from build123d import *

# Parameters (mm, degrees)
SKETCH1_W                  = 173.0375
SKETCH1_H                  = 114.3
BOSS_EXTRUDE1_DEPTH        = 3.175
SKETCH3_R                  = 3.175
SKETCH3_R_2                = 3.7703125
CUT_EXTRUDE1_DEPTH         = 149.360729792
F_6_CLEARANCE_HOLE1_D      = 4.3053
F_3_0_213_DIAMETER_HOLE1_D = 5.4102
F_1_4_CLEARANCE_HOLE1_D    = 7.14248
CUT_EXTRUDE5_REACH         = 150.361
SKETCH16_R                 = 1.190625
CUT_EXTRUDE6_DEPTH         = 149.360729792
FILLET5_R                  = 3.175
FILLET6_R                  = 3.175
FILLET7_R                  = 2.54


with BuildPart() as part:
    # Sketch1 → Boss-Extrude1 (new body)
    with BuildSketch(Plane.XY):
        with Locations((25.118, -40.513)):
            Rectangle(SKETCH1_W, SKETCH1_H)
    extrude(amount=BOSS_EXTRUDE1_DEPTH)

    # Sketch3 → Cut-Extrude1 (cut, through all)
    with BuildSketch(Plane.XY.offset(3.175)):
        with Locations((100.302, -26.543)):
            Circle(SKETCH3_R)
        with Locations((99.413, -51.6255)):
            Circle(SKETCH3_R_2)
        with Locations((-47.907, -51.6255)):
            Circle(SKETCH3_R_2)
        with Locations((-47.907, -6.5405)):
            Circle(SKETCH3_R_2)
    extrude(amount=-CUT_EXTRUDE1_DEPTH, mode=Mode.SUBTRACT)

    # #6 Clearance Hole1 (through all)
    with Locations(Plane.XY.offset(3.175)):
        with Locations((18.387, 10.287), (-56.162, -40.894), (106.398, -40.894), (18.387, -91.313)):
            Hole(F_6_CLEARANCE_HOLE1_D / 2)

    # #3 (0.213) Diameter Hole1 (through all)
    with Locations(Plane(origin=(18.387, 10.287, 3.175), x_dir=(1, 0, 0), z_dir=(0, 0, 1))):
        with Locations((0, 0), (-74.549, -51.181), (0, -101.6), (88.011, -51.181)):
            Hole(F_3_0_213_DIAMETER_HOLE1_D / 2)

    # 1/4 Clearance Hole1 (through all)
    with Locations(Plane(origin=(0, 0, 0), x_dir=(-1, 0, 0), z_dir=(0, 0, -1))):
        with Locations((-102.7785, 10.287), (52.5425, 10.287)):
            Hole(F_1_4_CLEARANCE_HOLE1_D / 2)

    # Sketch16 → Cut-Extrude5 (cut, up to next)
    with BuildSketch(Plane(origin=(0, 0, 0), x_dir=(-1, 0, 0), z_dir=(0, 0, -1)), mode=Mode.PRIVATE) as cut_extrude5_sk1:
        with Locations((-98.142490655, -57.489441166)):
            Circle(SKETCH16_R)
    cut_extrude5_tool1 = extrude(cut_extrude5_sk1.sketch, amount=-CUT_EXTRUDE5_REACH, mode=Mode.PRIVATE) & part.part
    # Sketch16 → Cut-Extrude5 (cut, up to next)
    with BuildSketch(Plane(origin=(0, 0, 0), x_dir=(-1, 0, 0), z_dir=(0, 0, -1)), mode=Mode.PRIVATE) as cut_extrude5_sk2:
        with Locations((49.177509345, -57.489441166)):
            Circle(SKETCH16_R)
    cut_extrude5_tool2 = extrude(cut_extrude5_sk2.sketch, amount=-CUT_EXTRUDE5_REACH, mode=Mode.PRIVATE) & part.part
    # Sketch16 → Cut-Extrude5 (cut, up to next)
    with BuildSketch(Plane(origin=(0, 0, 0), x_dir=(-1, 0, 0), z_dir=(0, 0, -1)), mode=Mode.PRIVATE) as cut_extrude5_sk3:
        with Locations((49.177509345, -12.404441166)):
            Circle(SKETCH16_R)
    cut_extrude5_tool3 = extrude(cut_extrude5_sk3.sketch, amount=-CUT_EXTRUDE5_REACH, mode=Mode.PRIVATE) & part.part
    add(cut_extrude5_tool1.solids().sort_by_distance((98.142491, -57.489441, 0))[0], mode=Mode.SUBTRACT)
    add(cut_extrude5_tool2.solids().sort_by_distance((-49.177509, -57.489441, 0))[0], mode=Mode.SUBTRACT)
    add(cut_extrude5_tool3.solids().sort_by_distance((-49.177509, -12.404441, 0))[0], mode=Mode.SUBTRACT)

    # Sketch17 → Cut-Extrude6 (cut, through all)
    with BuildSketch(Plane(origin=(0, 0, 0), x_dir=(-1, 0, 0), z_dir=(0, 0, -1))):
        Polygon((-89.41175, 10.287), (-59.68051, 10.287), (-59.68051, 14.25702), (-52.53549, 14.25702), (-52.53549, 10.287), (-34.28051, 10.287), (-34.28051, 14.25702), (-27.13549, 14.25702), (-27.13549, 10.287), (-24.737, 10.287), (-24.737, 5.5245), (-12.037, 5.5245), (-12.037, 10.287), (42.35075, 10.287), (42.35075, 5.5245), (48.70075, 5.5245), (48.70075, 0.762), (55.05075, 0.762), (55.05075, -36.1315), (48.2245, -36.1315), (48.2245, -45.26026), (56.63825, -45.26026), (56.63825, -91.313), (22.39451, -91.313), (22.39451, -94.488), (15.24949, -94.488), (15.24949, -91.313), (-12.037, -91.313), (-12.037, -86.5505), (-24.737, -86.5505), (-24.737, -91.313), (-70.36175, -91.313), (-70.36175, -94.488), (-92.58675, -94.488), (-92.58675, -89.7255), (-106.87425, -89.7255), (-106.87425, -45.26026), (-100.048, -45.26026), (-100.048, -36.1315), (-106.87425, -36.1315), (-106.87425, -28.194), (-109.22375, -28.194), (-109.22375, -23.4315), (-106.87425, -23.4315), (-106.87425, 0), (-99.72923, 0), (-99.72923, 3.175), (-89.41175, 3.175), align=None)
    extrude(amount=-CUT_EXTRUDE6_DEPTH, mode=Mode.SUBTRACT)

    # Fillet5
    # the kernel refuses this fillet: 3.175 mm, written as the material it adds along each edge
    with BuildSketch(Plane(origin=(106.87425, 0, 0), x_dir=(0, -1, 0), z_dir=(0, 0, 1)), Plane(origin=(106.87425, -45.26026, 0), x_dir=(0, -1, 0), z_dir=(0, 0, 1)), Plane(origin=(106.87425, -36.1315, 0), x_dir=(-1, 0, 0), z_dir=(0, 0, 1)), Plane(origin=(106.87425, -89.7255, 0), x_dir=(-1, 0, 0), z_dir=(0, 0, 1)), Plane(origin=(92.58675, -94.488, 0), x_dir=(-1, 0, 0), z_dir=(0, 0, 1)), Plane(origin=(70.36175, -94.488, 0), x_dir=(0, 1, 0), z_dir=(0, 0, 1)), Plane(origin=(24.737, -91.313, 0), x_dir=(0, 1, 0), z_dir=(0, 0, 1)), Plane(origin=(12.037, -91.313, 0), x_dir=(-1, 0, 0), z_dir=(0, 0, 1)), Plane(origin=(-15.24949, -94.488, 0), x_dir=(-1, 0, 0), z_dir=(0, 0, 1)), Plane(origin=(-22.39451, -94.488, 0), x_dir=(0, 1, 0), z_dir=(0, 0, 1)), Plane(origin=(-56.63825, -91.313, 0), x_dir=(0, 1, 0), z_dir=(0, 0, 1)), Plane(origin=(-55.05075, -36.1315, 0), x_dir=(0, 1, 0), z_dir=(0, 0, 1)), Plane(origin=(-56.63825, -45.26026, 0), x_dir=(1, 0, 0), z_dir=(0, 0, 1)), Plane(origin=(-55.05075, 0.762, 0), x_dir=(1, 0, 0), z_dir=(0, 0, 1)), Plane(origin=(-48.70075, 5.5245, 0), x_dir=(1, 0, 0), z_dir=(0, 0, 1)), Plane(origin=(-42.35075, 10.287, 0), x_dir=(1, 0, 0), z_dir=(0, 0, 1)), Plane(origin=(12.037, 10.287, 0), x_dir=(0, -1, 0), z_dir=(0, 0, 1)), Plane(origin=(34.28051, 14.25702, 0), x_dir=(0, -1, 0), z_dir=(0, 0, 1)), Plane(origin=(27.13549, 14.25702, 0), x_dir=(1, 0, 0), z_dir=(0, 0, 1)), Plane(origin=(52.53549, 14.25702, 0), x_dir=(1, 0, 0), z_dir=(0, 0, 1)), Plane(origin=(59.68051, 14.25702, 0), x_dir=(0, -1, 0), z_dir=(0, 0, 1))) as fillet5_piece_1:
        with BuildLine():
            CenterArc((FILLET5_R, -FILLET5_R), FILLET5_R, 90, 90)
            Line((0, -FILLET5_R), (-FILLET5_R * 0.02, -FILLET5_R))
            Line((-FILLET5_R * 0.02, -FILLET5_R), (-FILLET5_R * 0.02, FILLET5_R * 0.02))
            Line((-FILLET5_R * 0.02, FILLET5_R * 0.02), (FILLET5_R, FILLET5_R * 0.02))
            Line((FILLET5_R, FILLET5_R * 0.02), (FILLET5_R, 0))
        make_face()
    extrude(amount=3.175)
    with BuildSketch(Plane(origin=(24.737, 10.287, 0), x_dir=(1, 0, 0), z_dir=(0, 0, 1))) as fillet5_piece_2:
        with BuildLine():
            CenterArc((3.175, -3.07858039), FILLET5_R, 104.15642815, 75.84357185)
            Line((0, -3.07858039), (-0.0635, -3.07858039))
            Line((-0.0635, -3.07858039), (-0.0635, 0))
            Line((-0.0635, 0), (0, 0.0635))
            ThreePointArc((0, 0.0635), (1.199245, 0.0635), (2.3829598, 0.061571608))
            Line((2.3829598, 0.061571608), (2.39849, 0))
        make_face()
    extrude(amount=3.175)
    with BuildSketch(Plane(origin=(89.41175, 10.287, 0), x_dir=(-1, 0, 0), z_dir=(0, 0, 1))) as fillet5_piece_3:
        with BuildLine():
            CenterArc((FILLET5_R, FILLET5_R), FILLET5_R, 180, 90)
            Line((0, FILLET5_R), (-FILLET5_R * 0.02, FILLET5_R))
            Line((-FILLET5_R * 0.02, FILLET5_R), (-FILLET5_R * 0.02, -FILLET5_R * 0.02))
            Line((-FILLET5_R * 0.02, -FILLET5_R * 0.02), (FILLET5_R, -FILLET5_R * 0.02))
            Line((FILLET5_R, -FILLET5_R * 0.02), (FILLET5_R, 0))
        make_face()
    extrude(amount=3.175)
    # the kernel refuses this fillet: 3.175 mm, written as the material it takes off along each edge
    with BuildSketch(Plane(origin=(99.72923, 0, -7.9375), x_dir=(1, 0, 0), z_dir=(0, 0, 1)), Plane(origin=(89.41175, 3.175, -7.9375), x_dir=(1, 0, 0), z_dir=(0, 0, 1))) as fillet5_2_piece_1:
        with BuildLine():
            CenterArc((FILLET5_R, FILLET5_R), FILLET5_R, 180, 90)
            Line((0, FILLET5_R), (-FILLET5_R * 0.02, FILLET5_R))
            Line((-FILLET5_R * 0.02, FILLET5_R), (-FILLET5_R * 0.02, -FILLET5_R * 0.02))
            Line((-FILLET5_R * 0.02, -FILLET5_R * 0.02), (FILLET5_R, -FILLET5_R * 0.02))
            Line((FILLET5_R, -FILLET5_R * 0.02), (FILLET5_R, 0))
        make_face()
    extrude(amount=19.05, mode=Mode.SUBTRACT)
    with BuildSketch(Plane(origin=(106.87425, -23.4315, -7.664518392), x_dir=(1, 0, 0), z_dir=(0, 0, 1))) as fillet5_2_piece_2:
        with BuildLine():
            CenterArc((3.175, 3.065807357), FILLET5_R, 180, 74.929937855)
            Line((0, 3.065807357), (-0.0635, 3.065807357))
            Line((-0.0635, 3.065807357), (-0.0635, 0))
            Line((-0.0635, 0), (0, -0.0635))
            ThreePointArc((0, -0.0635), (1.17475, -0.0635), (2.33299, -0.061316147))
            Line((2.33299, -0.061316147), (2.3495, 0))
        make_face()
    extrude(amount=18.504036785, mode=Mode.SUBTRACT)
    with BuildSketch(Plane(origin=(106.87425, -28.194, -7.664518392), x_dir=(0, -1, 0), z_dir=(0, 0, 1))) as fillet5_2_piece_3:
        with BuildLine():
            CenterArc((3.065807357, 3.175), FILLET5_R, 195.070062145, 74.929937855)
            Line((0, 2.3495), (-0.061316147, 2.33299))
            ThreePointArc((-0.061316147, 2.33299), (-0.0635, 1.17475), (-0.0635, 0))
            Line((-0.0635, 0), (0, -0.0635))
            Line((0, -0.0635), (3.065807357, -0.0635))
            Line((3.065807357, -0.0635), (3.065807357, 0))
        make_face()
    extrude(amount=18.504036785, mode=Mode.SUBTRACT)

    # Fillet6
    fillet6_edges = [part.edges().sort_by_distance(p)[0] for p in [
        (99.72923, 3.175, 1.5875),
        (59.68051, 10.287, 1.5875),
        (52.53549, 10.287, 1.5875),
        (34.28051, 10.287, 1.5875),
        (27.13549, 10.287, 1.5875),
        (24.737, 5.5245, 1.5875),
        (12.037, 5.5245, 1.5875),
        (-42.35075, 5.5245, 1.5875),
        (-48.70075, 0.762, 1.5875),
        (-48.2245, -36.1315, 1.5875),
        (-48.2245, -45.26026, 1.5875),
        (-22.39451, -91.313, 1.5875),
        (-15.24949, -91.313, 1.5875),
        (12.037, -86.5505, 1.5875),
        (24.737, -86.5505, 1.5875),
        (70.36175, -91.313, 1.5875),
        (92.58675, -89.7255, 1.5875),
        (100.048, -45.26026, 1.5875),
        (100.048, -36.1315, 1.5875),
        (109.22375, -28.194, 1.5875),
        (109.22375, -23.4315, 1.5875),
    ]]
    fillet(fillet6_edges, radius=FILLET6_R)

    # Fillet7
    fillet7_edges = [part.edges().sort_by_distance(p)[0] for p in [
        (-61.40075, 16.637, 1.5875),
        (111.63675, 16.637, 1.5875),
        (111.63675, -97.663, 1.5875),
        (-61.40075, -97.663, 1.5875),
    ]]
    fillet(fillet7_edges, radius=FILLET7_R)


solid = part.part
Build history of the part. All positions in model axes, mm. Coordinates: 2 decimals unless noted, no trailing zeros. Write each loop counter-clockwise with the first axis right and the second up, starting at its lowest first coordinate (ties: lowest second). Pieces come first, ordered by that corner, then holes. Notation, with made-up numbers: (2, 16) -> (54, 16) arc R36 cw to (54, 50) -> close; hole circle Ø3 at (14, 56.5). An arc over 180 degrees is marked (long way). Use CSV: the item, a comma, the result in double quotes. Start each with the question number.
Q1. Cut at A-A, the plane y = -76. List the corners of the cut face in (x, z) (3 decimals).
Q2. Drill centre lines: probe 1 along Y at (x, z) = (81.5, 0.2); probe 2 along X at (y, z) = (-17, 1); probe 3 along Y at (x, z) = (-45, 2.6). Where is each one in solid material? Low to high.
Q3. Cut at B-B, the plane x = -7. List the corners of the cut face in (y, z) (3 decimals), then the cut area to 3 significant figures.
Q4. Pull direction X, two halves, no side cores. Call faces 1 (the flat face through (24, -97.663, 2)), 2 (the cylindrical face through (105.969, -46.215, 1.565)), 3 (the flat face through (-39, -91.313, 2)): released by +X, released by -X, zero draft, split by the parting line, or undercut.
Q5. Flat gauge pin, fed straight in: pin 1 Ø6 at (x, y) = (18.387, 10.287) entering from +Z (3 decimals). Where does the tip first touch, or does it go through?
Q6. Cut at C-C, the plane z = 1.9. State how many separate pieces and enclosed holes the cut face has, then the cut area to 3 significant figures.
Checked values:
1,outline,"(-61.401, 0) -> (-56.638, 0) -> (-56.638, 3.175) -> (-61.401, 3.175) -> close; (106.874, 0) -> (111.637, 0) -> (111.637, 3.175) -> (106.874, 3.175) -> close"
2,probe 1,"y = -97.66 to -94.49, 10.29 to 16.64"
2,probe 2,"x = -61.4 to -55.05, 106.87 to 111.64"
2,probe 3,"y = -97.66 to -91.31, 5.54 to 16.64"
3,outline,"(-97.663, 0) -> (-91.313, 0) -> (-91.313, 3.175) -> (-97.663, 3.175) -> close; (10.287, 0) -> (16.637, 0) -> (16.637, 3.175) -> (10.287, 3.175) -> close"
3,area,"40.3 mm²"
4,face 1,"zero draft"
4,face 2,"undercut"
4,face 3,"undercut"
5,pin 1,"stops at z = 3.175"
6,separate pieces,"1"
6,enclosed holes,"7"
6,area,"3,440 mm²"
